```python
from build123d import *

# Parameters (mm, degrees)
SKETCH1_R           = 50.546
SKETCH1_R_2         = 48.006
BOSS_EXTRUDE1_DEPTH = 145.8595
SKETCH2_R           = 50.546
BOSS_EXTRUDE2_DEPTH = 1.9812
SKETCH3_R           = 14.605
CUT_EXTRUDE1_DEPTH  = 161.657279458


with BuildPart() as part:
    # Sketch1 → Boss-Extrude1 (new body)
    with BuildSketch(Plane(origin=(0, 0, 0), x_dir=(1, 0, 0), z_dir=(0, 1, 0))):
        with Locations(Location((0, 0, 0), (0, 0, 270))):
            Circle(SKETCH1_R)
        with Locations(Location((0, 0, 0), (0, 0, 270))):
            Circle(SKETCH1_R_2, mode=Mode.SUBTRACT)
    extrude(amount=BOSS_EXTRUDE1_DEPTH)

    # Sketch2 → Boss-Extrude2 (add)
    with BuildSketch(Plane.XZ):
        with Locations(Location((0, 0, 0), (0, 0, 90))):
            Circle(SKETCH2_R)
    extrude(amount=-BOSS_EXTRUDE2_DEPTH)

    # Sketch3 → Cut-Extrude1 (cut, through all)
    with BuildSketch(Plane(origin=(0, 1.9812, 0), x_dir=(-1, 0, 0), z_dir=(0, 1, 0))):
        with Locations(Location((0, 28.575, 0), (0, 0, 90))):
            Circle(SKETCH3_R)
    extrude(amount=-CUT_EXTRUDE1_DEPTH, mode=Mode.SUBTRACT)


solid = part.part
```
Check sheet for the modelled part. Datum: model origin and axes. Units: mm. A direction names the side the tool comes from. Round coordinates to 2 decimals unless told otherwise and drop trailing zeros. Write each loop counter-clockwise with the first axis right and the second up, starting at its lowest first coordinate (ties: lowest second). Pieces come first, ordered by that corner, then holes. Notation, with made-up numbers: M 89,-31.75 L 121,-31.75 A31 ccw 121,-2.75 Z; hole C -10,-20 d2. An arc over 180 degrees is marked long. Write item = value, one per line. Start each with the question number.
1. Section check B-B, the plane z = 27.5. Record the cut outline in (x, y), then the cut area to 3 significant figures.
2. Scan lines: line 1 (X direction, y = 19, z = 0.5); line 2 (Y direction, x = 1.5, z = 12); line 3 (X direction, y = 131.5, z = -11.5). Record each from-to range of solid material in increasing order. Write a range as [from, to].
3. Section check A-A, the plane x = 0. Record the cut outline in (y, z), then the cut area to 3 significant figures.
4. Release check for a two-part mould opening along X. For faces 1 (the flat face through (-18, 145.86, 45)), 2 (the cylindrical face through (0.642, 1.004, 13.984)), 3 (the cylindrical face through (-19.36, 71.91, 46.69)), 4 (the cylindrical face through (-46.864, 72.913, -10.407)) record: pulls with the +X half, pulls with the -X half, needs draft (parallel to the pull), parting line crosses it, or undercut.
5. Section check D-D, the plane y = 108. Record the cut outline in (x, z).
6. Section check C-C, the plane z = 0. Record the cut outline in (x, y).
7. Tool access check on faces 5 (the flat face through (-1, 1.981, -1)), 6 (the flat face through (1, 0, -1)). Record the directions out of +Z, -Z, +X, -X, +Y, -Y that give a thin tool (end or side, any length) a straight path to the whole face; none if there is none.
8. Gauge pin test, flat ends, axial feed: pin 1 (1 mm diameter, centred on y = 34.5, z = -19, fed in from +X); pin 2 (5 mm diameter, centred on x = 20.5, y = 64, fed in from -Z); pin 3 (8 mm diameter, centred on x = -3.5, z = -30, fed in from -Y); pin 4 (3 mm diameter, centred on x = -14, y = 109.5, fed in from +Z). Record the tip position at first contact, or that the pin passes through.
Results found:
q1.outline = M -42.41,0 L -14.57,0 L -14.57,1.98 L -39.35,1.98 L -39.35,145.86 L -42.41,145.86 Z; M 14.57,0 L 42.41,0 L 42.41,145.86 L 39.35,145.86 L 39.35,1.98 L 14.57,1.98 Z
q1.area = 991 mm^2
q2.line_1 = [-50.54, -48], [48, 50.54]
q2.line_2 = [0, 1.98]
q2.line_3 = [-49.22, -46.61], [46.61, 49.22]
q3.outline = M 0,-50.55 L 145.86,-50.55 L 145.86,-48.01 L 1.98,-48.01 L 1.98,13.97 L 0,13.97 Z; M 0,43.18 L 1.98,43.18 L 1.98,48.01 L 145.86,48.01 L 145.86,50.55 L 0,50.55 Z
q3.area = 873 mm^2
q4.face_1 = needs draft
q4.face_2 = undercut
q4.face_3 = parting line crosses it
q4.face_4 = undercut
q5.outline = C 0,0 d101.09; hole C 0,0 d96.01
q6.outline = M -50.55,0 L 50.55,0 L 50.55,145.86 L 48.01,145.86 L 48.01,1.98 L -48.01,1.98 L -48.01,145.86 L -50.55,145.86 Z
q7.face_5 = +Y
q7.face_6 = +Z, -Z, +X, -X, -Y
q8.pin_1 = 47.04
q8.pin_2 = -47.23
q8.pin_3 = 0
q8.pin_4 = 48.98
